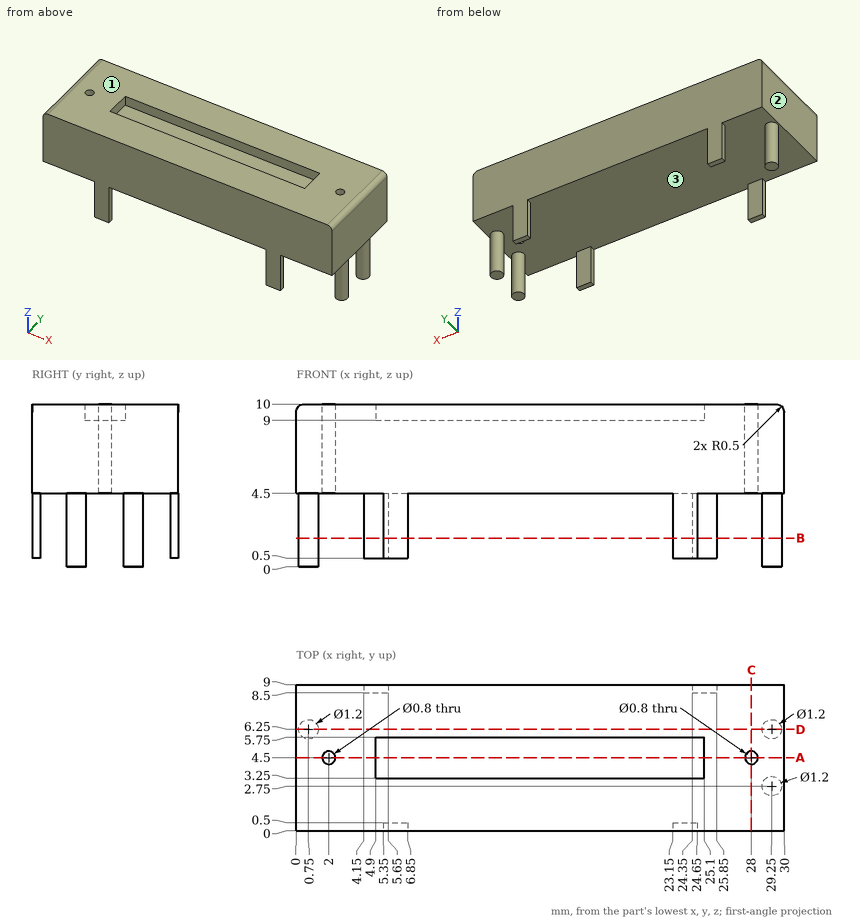
Print and shaded views of the part. All mm, measured from the part's lowest x, y and z. Coordinates: 2 decimals unless noted, no trailing zeros. Write each loop counter-clockwise with the first axis right and the second up, starting at its lowest first coordinate (ties: lowest second). Pieces come first, ordered by that corner, then holes.
(1) Flat gauge pins, fed straight in: pin 1 (1 mm diameter, centred on x = 16, y = 5.5, fed in from -Z); pin 2 (1 mm diameter, centred on x = 25.5, z = 3, fed in from -Y); pin 3 (0.6 mm diameter, centred on y = 0, z = 3, fed in from +X). Where does each tip first touch, or does it go through?
(2) Cut at D-D, the plane y = 6.25. List the corners of the cut face in (x, z).
(3) Cut at C-C, the plane x = 28. List the corners of the cut face in (y, z), and give its area (3 significant figures).
(4) Cut at A-A, the plane y = 4.5. List the corners of the cut face in (x, z), and give its area (3 significant figures).
(5) Two-plate mould, pull along X, no slides. Class the marked faces 1, 2 and 3: +X half, -X half, draft (parallel to the pull), parting line (faces both ways), or undercut.
(6) Cut at B-B, the plane z = 1.75. List the corners of the cut face in (x, y), and give its area (3 significant figures).
(7) Drill centre lines: probe 1 along Y at (x, z) = (2, 6.2); probe 2 along Y at (x, z) = (23.5, 4.25); probe 3 along Z at (x, y) = (16.5, 2). Where is each one in solid material? Low to high.
Geometry says:
1. pin 1: stops at z = 4.5
1. pin 2: stops at y = 8.5
1. pin 3: stops at x = 24.65
2. outline: (0, 4.5) - (0.15, 4.5) - (0.15, 0) - (1.35, 0) - (1.35, 4.5) - (28.65, 4.5) - (28.65, 0) - (29.85, 0) - (29.85, 4.5) - (30, 4.5) - (30, 9.5) arc R0.5 ccw to (29.5, 10) - (0.5, 10) arc R0.5 ccw to (0, 9.5) - close
3. outline: (0, 4.5) - (4.1, 4.5) - (4.1, 10) - (0, 10) - close; (4.9, 4.5) - (9, 4.5) - (9, 10) - (4.9, 10) - close
3. area: 45.1 mm2
4. outline: (0, 4.5) - (1.6, 4.5) - (1.6, 10) - (0.5, 10) arc R0.5 ccw to (0, 9.5) - close; (2.4, 4.5) - (27.6, 4.5) - (27.6, 10) - (25.1, 10) - (25.1, 9) - (4.9, 9) - (4.9, 10) - (2.4, 10) - close; (28.4, 4.5) - (30, 4.5) - (30, 9.5) arc R0.5 ccw to (29.5, 10) - (28.4, 10) - close
4. area: 136 mm2
5. face 1: draft
5. face 2: -X half
5. face 3: undercut
6. outline: circle Ø1.2 at (0.75, 6.25); (4.15, 8.5) - (5.65, 8.5) - (5.65, 9) - (4.15, 9) - close; (5.35, 0) - (6.85, 0) - (6.85, 0.5) - (5.35, 0.5) - close; (23.15, 0) - (24.65, 0) - (24.65, 0.5) - (23.15, 0.5) - close; (24.35, 8.5) - (25.85, 8.5) - (25.85, 9) - (24.35, 9) - close; circle Ø1.2 at (29.25, 2.75); circle Ø1.2 at (29.25, 6.25)
6. area: 6.39 mm2
7. probe 1: y = 0 to 4.1, 4.9 to 9
7. probe 2: y = 0 to 0.5
7. probe 3: z = 4.5 to 10
